Can you work these out from the model? Positions are in its coordinate system, mm. A direction names the side the tool comes from. Give positions to 0.01 mm unless a question says otherwise; leave off trailing zeros. Loops run counter-clockwise (first coordinate to the right, second up) from the corner with the lowest first, then second, coordinate; pieces in that order, holes last. Notation, with made-up numbers: (34.25, 80.5) -> (80.25, 80.5) arc R21 cw to (80.25, 119.5) -> close; hole circle Ø5 at (14, 87). An arc over 180 degrees is marked (long way). Return JSON: item names as keys, results as strings. Group by question number.
Q1. Suppose I cut it at B-B, the plane x = -12.7. Please give me the cut outline in (y, z) (3 decimals).
Q2. Will these pins go through, and if not, where does the flat tip stop? pin 1 (12.5 mm diameter, centred on x = -114.3, z = 25.4, fed in from +Y); pin 2 (10 mm diameter, centred on y = 11, z = 34.5, fed in from +X) (3 decimals); pin 3 (6 mm diameter, centred on y = 17.5, z = 41.5, fed in from -X); pin 4 (2.5 mm diameter, centred on y = 13.5, z = 50, fed in from +X).
Q3. Suppose I cut it at C-C, the plane x = -63.5. Please give me the cut outline in (y, z) (3 decimals), and give its area (3 significant figures).
Q4. I need wall thicknesses on line 1 along Y through (x, z) = (-72.5, 12.5) (3 decimals); line 2 along Z through (x, y) = (-115.5, 17.5) (3 decimals); line 3 along X through (y, z) = (1.1, 38.1) (3 decimals). Which ranges of each line are inside material? Lowest first, please. Write a range as [from, to].
Q5. Thinking about a two-plate mould opening in Y: for faces 1 (the flat face through (-31.75, 13, 49)), 2 (the cylindrical face through (-65.646, 1.565, 10.36)), which applies, pulls with the +Y half, pulls with the -Y half, needs draft (parallel to the pull), parting line crosses it, or undercut?
Q6. Suppose I cut it at A-A, the plane z = 12.7. Please give me the cut outline in (x, y) (3 decimals), and give its area (3 significant figures).
Q7. Which directions (+Z, -Z, +X, -X, +Y, -Y) give clear straight access to the entire face, cutting with the end or side of a thin tool? Please do faces 3 (the flat face through (-65, 13, 47.625)), 4 (the flat face through (-114, 22.225, 20)), 5 (the flat face through (-127, 2, 27)), 6 (the flat face through (-31.75, 13, 2)), 7 (the flat face through (0, 24, 25)).
Q8. Suppose I cut it at D-D, the plane z = 38.1. Please give me the cut outline in (x, y) (3 decimals).
Autodesk Inventor part; units mm, degrees
ref_plane "YZ Plane" through (0, 0, 0) normal (1, 0, 0) x (0, 1, 0)
ref_plane "XZ Plane" through (0, 0, 0) normal (0, 1, 0) x (-1, 0, 0)
ref_plane "XY Plane" through (0, 0, 0) normal (0, 0, 1) x (1, 0, 0)
sketch "Sketch1" plane through (0, 0, 0) normal (0, 0, 1) x (1, 0, 0)
  line L0 (0, 0) -> (-127, 0)
  line L1 (-127, 0) -> (-127, 25.4)
  line L2 (-127, 25.4) -> (0, 25.4)
  line L3 (0, 0) -> (0, 3.175)
  line L4 (0, 3.175) -> (-98.425, 3.175)
  line L5 (-98.425, 3.175) -> (-98.425, 22.225)
  line L6 (-98.425, 22.225) -> (0, 22.225)
  line L7 (0, 22.225) -> (0, 25.4)
  dimension "d0" = 127
  dimension "d1" = 25.4
  dimension "d2" = 3.175
  dimension "d3" = 98.425
  dimension "d4" = 19.05
extrude "Extrusion1" add sketch "Sketch1" along normal blind 50.8
sketch "Sketch2" plane through (-127, 25.4, 0) normal (0, 1, 0) x (1, 0, 0)
  circle A0 centre (114.3, -38.1) radius 3.175
  line L0 (127, 0) -> (127, -50.8)
  line L1 (127, -50.8) -> (0, -50.8)
  line L2 (0, -50.8) -> (127, -50.8)
  line L3 (0, -50.8) -> (95.25, -50.8)
  line L4 (95.25, -50.8) -> (95.25, -47.625)
  line L5 (95.25, -47.625) -> (0, -47.625)
  line L6 (0, -47.625) -> (0, -50.8)
  line L7 (127, 0) -> (0, 0)
  line L8 (0, -3.175) -> (95.25, -3.175)
  line L9 (95.25, -3.175) -> (95.25, 0)
  line L10 (95.25, 0) -> (0, 0)
  line L11 (0, 0) -> (0, -3.175)
  circle A1 centre (12.7, -25.4) radius 4.7625
  line L12 (0, 0) -> (0, -50.8)
  dimension "d7" = 6.35
  dimension "d8" = 12.7
  dimension "d9" = 12.7
  dimension "d12" = 31.75
  dimension "d13" = 3.175
  dimension "d19" = 9.525
  dimension "d20" = 12.7
  dimension "d21" = 25.4
extrude "Extrusion2" cut sketch "Sketch2" against normal blind 50.8 contours A0 | A1
extrude "Extrusion3" add sketch "Sketch2" against normal blind 25.4 contours L9 L8 L11 L7 | L1 L6 L5 L4
sketch "Sketch3" plane through (-127, 0, 0) normal (-1, 0, 0) x (0, 0, 1)
  line L0 (3.175, 22.225) -> (3.175, 3.175)
  line L1 (0, 22.225) -> (50.8, 22.225)
  line L2 (3.175, 3.175) -> (47.625, 3.175)
  line L3 (47.625, 3.175) -> (47.625, 22.225)
  line L4 (47.625, 22.225) -> (3.175, 22.225)
  line L5 (3.175, 22.225) -> (3.175, 3.175)
  point P0 (0, 0)
  dimension "d16" = 44.45
extrude "Extrusion4" cut sketch "Sketch3" against normal blind 25.4
sketch "Sketch4" plane through (-127, 25.4, 50.8) normal (0, 1, 0) x (1, 0, 0)
  line L0 (0, 50.8) -> (127, 50.8)
  line L1 (127, 0) -> (0, 0)
  line L2 (0, 50.8) -> (0, 0)
  point P0 (38.1, 12.7)
  point P1 (63.5, 38.1)
  dimension "d22" = 12.7
  dimension "d23" = 12.7
  dimension "d24" = 38.1
  dimension "d25" = 63.5
hole "Hole1" at (-88.9, 25.4, 38.1) at (-63.5, 25.4, 12.7) direction (0, -1, 0) diameter 6.35 end through all
properties part number "15102898-16-P-0203" material "Aluminum 6061"
Ans:
{
 "1": {"outline": "(0, 0) -> (3.175, 0) -> (3.175, 34.925) -> (0, 34.925) -> close; (0, 41.275) -> (3.175, 41.275) -> (3.175, 50.8) -> (0, 50.8) -> close; (22.225, 0) -> (25.4, 0) -> (25.4, 34.925) -> (22.225, 34.925) -> close; (22.225, 41.275) -> (25.4, 41.275) -> (25.4, 50.8) -> (22.225, 50.8) -> close"},
 "2": {"pin 1": "stops at y = 25.4", "pin 2": "stops at x = -98.425", "pin 3": "stops at x = -101.6", "pin 4": "stops at x = -31.75"},
 "3": {"outline": "(0, 0) -> (25.4, 0) -> (25.4, 9.525) -> (22.225, 9.525) -> (22.225, 3.175) -> (3.175, 3.175) -> (3.175, 9.525) -> (0, 9.525) -> close; (0, 15.875) -> (3.175, 15.875) -> (3.175, 47.625) -> (22.225, 47.625) -> (22.225, 15.875) -> (25.4, 15.875) -> (25.4, 50.8) -> (0, 50.8) -> close", "area": "403 mm^2"},
 "4": {"line 1": "y = [0, 3.175], [22.225, 25.4]", "line 2": "z = [0, 3.175], [47.625, 50.8]", "line 3": "x = [-127, -92.075], [-85.725, -15.875], [-9.525, 0]"},
 "5": {"face 1": "undercut", "face 2": "needs draft"},
 "6": {"outline": "(-127, 0) -> (-66.675, 0) -> (-66.675, 3.175) -> (-98.425, 3.175) -> (-98.425, 22.225) -> (-66.675, 22.225) -> (-66.675, 25.4) -> (-127, 25.4) -> (-127, 22.225) -> (-101.6, 22.225) -> (-101.6, 3.175) -> (-127, 3.175) -> close; (-60.325, 0) -> (0, 0) -> (0, 3.175) -> (-60.325, 3.175) -> close; (-60.325, 22.225) -> (0, 22.225) -> (0, 25.4) -> (-60.325, 25.4) -> close", "area": "827 mm^2"},
 "7": {"face 3": "+X", "face 4": "-X", "face 5": "+Z, -Z, -X, +Y, -Y", "face 6": "+Z, -Z, +X", "face 7": "+Z, -Z, +X, +Y, -Y"},
 "8": {"outline": "(-127, 0) -> (-92.075, 0) -> (-92.075, 3.175) -> (-98.425, 3.175) -> (-98.425, 22.225) -> (-92.075, 22.225) -> (-92.075, 25.4) -> (-127, 25.4) -> (-127, 22.225) -> (-101.6, 22.225) -> (-101.6, 3.175) -> (-127, 3.175) -> close; (-85.725, 0) -> (-15.875, 0) -> (-15.875, 3.175) -> (-85.725, 3.175) -> close; (-85.725, 22.225) -> (-15.875, 22.225) -> (-15.875, 25.4) -> (-85.725, 25.4) -> close; (-9.525, 0) -> (0, 0) -> (0, 3.175) -> (-9.525, 3.175) -> close; (-9.525, 22.225) -> (0, 22.225) -> (0, 25.4) -> (-9.525, 25.4) -> close"}
}
